Design review of the part built by this model. Coordinates are the model's own, in mm. Face numbers are marked on the shaded views. A direction names the side the tool comes from. Give positions to 0.01 mm unless a question says otherwise; leave off trailing zeros. Order: outer loops, then holes, each group sorted by start corner. A loop starts at its lowest first (then second) coordinate and runs counter-clockwise, first axis right, second up. Notation, with made-up numbers: M -3,63.25 L 22,63.25 A29 ccw 22,94.25 Z; hole C -29.75,36 d11. An arc over 180 degrees is marked long. Answer as a JSON object with one key per item and string values.
from build123d import *

# Parameters (mm, degrees)
F0_W     = 50.8
F0_H     = 50.8
F0_W_2   = 25.4
F0_H_2   = 25.4
F1_DEPTH = 88.9
F2_W     = 65.903696
F2_H     = 43.18
F3_DEPTH = 50.8


with BuildPart() as f1:
    # F0 (on Right) → F1 (new body)
    with BuildSketch(Plane.YZ):
        with Locations((8.370453, -3.046589)):
            Rectangle(F0_W, F0_H)
        with Locations((6.725227, -5.875227)):
            Rectangle(F0_W_2, F0_H_2, mode=Mode.SUBTRACT)
    extrude(amount=F1_DEPTH)

    # F2 (on face) → F3 (cut)
    with BuildSketch(Plane(origin=(0, 33.770453, 0), x_dir=(-1, 0, 0), z_dir=(0, 1, 0))):
        with Locations((-43.497203, 0.763411)):
            Rectangle(F2_W, F2_H)
    extrude(amount=-F3_DEPTH, mode=Mode.SUBTRACT)


solid = f1.part
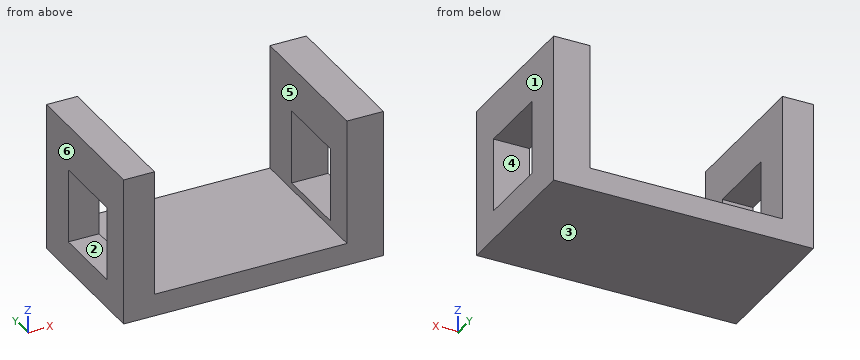
(1) We need section A-A (z = 5.5). Write out the cut boundary in (x, y), plus the area to 3 significant figures.
Checked values:
{"outline": "M 0,-17.03 L 10.55,-17.03 L 10.55,-5.97 L 0,-5.97 Z; M 0,19.43 L 10.55,19.43 L 10.55,33.77 L 0,33.77 Z; M 76.45,-17.03 L 88.9,-17.03 L 88.9,-5.97 L 76.45,-5.97 Z; M 76.45,19.43 L 88.9,19.43 L 88.9,33.77 L 76.45,33.77 Z", "area": "584 mm^2"}
(2) Draft analysis for pull direction Z (two halves, no side actions). For the marked faces 1, 2 and 3, state which applies: +Z half, -Z half, draft (parallel to the pull), parting line (faces both ways), or undercut.
Checked values:
{"face 1": "draft", "face 2": "undercut", "face 3": "-Z half"}
(3) Insertion check: pin 1 (6 mm diameter, centred on y = 4, z = -15.5, fed in from -X). The pin has a flat end and moves straight along its axis. Give the tip position at first contact, or say it passes through.
Checked values:
{"pin 1": "passes through"}
(4) We need section C-C (y = 7). Write out the cut boundary in (x, z).
Checked values:
{"outline": "M 0,-28.45 L 88.9,-28.45 L 88.9,-18.58 L 76.45,-18.58 L 76.45,-20.83 L 10.55,-20.83 L 10.55,-18.58 L 0,-18.58 Z; M 0,6.82 L 10.55,6.82 L 10.55,22.35 L 0,22.35 Z; M 76.45,6.82 L 88.9,6.82 L 88.9,22.35 L 76.45,22.35 Z"}
(5) We need section D-D (y = -9.5). Write out the cut boundary in (x, z).
Checked values:
{"outline": "M 0,-28.45 L 88.9,-28.45 L 88.9,22.35 L 76.45,22.35 L 76.45,-20.83 L 10.55,-20.83 L 10.55,22.35 L 0,22.35 Z"}
(6) Tool access review of the marked faces 4, 5 and 6: name each direction out of +Z, -Z, +X, -X, +Y, -Y from which nothing blocks a thin tool from reaching the whole face with its end or side.
Checked values:
{"face 4": "+X, -X", "face 5": "+Z, +Y, -Y", "face 6": "+Z, -Z, -X, +Y, -Y"}
(7) We need section B-B (x = 80.5). Write out the cut boundary in (y, z).
Checked values:
{"outline": "M -17.03,-28.45 L 33.77,-28.45 L 33.77,22.35 L -17.03,22.35 Z; hole M -5.97,-18.58 L 19.43,-18.58 L 19.43,6.82 L -5.97,6.82 Z"}
(8) To check wall thickness, follow L1, parallel to X at y = -9.5, z = 9.5; L2, parallel to Y at x = 5.5, z = -16.5; L3, parallel to Z at x = 30.5, y = 14. State the ranges of each line that lie inside material, in increasing order. Write a range as from..to.
Checked values:
{"L1": "x = 0..10.55, 76.45..88.9", "L2": "y = -17.03..-5.97, 19.43..33.77", "L3": "z = -28.45..-20.83"}
